Could you check a few things on this model? Use its own coordinates, in mm. Coordinates: 2 decimals unless noted, no trailing zeros. Loops run counter-clockwise (first coordinate to the right, second up) from the corner with the lowest first, then second, coordinate; pieces in that order, holes last. Notation, with made-up numbers: (-16.75, 58) - (21.25, 58) arc R24 ccw to (21.25, 83) - close; hole circle Ø7 at (14.25, 73). An arc over 180 degrees is marked (long way). Put each result on its own line as item: value. Start each with the question number.
```python
from build123d import *

# Parameters (mm, degrees)
F0_W     = 37
F0_H     = 56
F0_W_2   = 20
F0_H_2   = 20
F0_W_3   = 23
F0_H_3   = 23
F0_W_4   = 26
F0_H_4   = 18.5
F0_W_5   = 27
F0_H_5   = 3
F1_DEPTH = 1.5


with BuildPart() as f1:
    # F0 (on Top) → F1 (new body, symmetric)
    with BuildSketch(Plane.XY):
        with BuildLine():
            Line((-36.7347033552, 107.9341696352), (-246.7347033552, 107.9341696352))
            Line((-246.7347033552, 107.9341696352), (-246.7347033552, -140.0658303648))
            Line((-246.7347033552, -140.0658303648), (-36.7347033552, -140.0658303648))
            ThreePointArc((-36.7347033552, -140.0658303648), (-1.3793642959, -125.4211694242), (13.2652966448, -90.0658303648))
            Line((13.2652966448, -90.0658303648), (13.2652966448, 57.9341696352))
            ThreePointArc((13.2652966448, 57.9341696352), (-1.3793642959, 93.2895086945), (-36.7347033552, 107.9341696352))
        make_face()
        with Locations((-80.5683995187, -99.1663551629)):
            Rectangle(F0_W, F0_H, mode=Mode.SUBTRACT)
        with Locations((-43.9143308997, -91.0555796049)):
            Rectangle(F0_W_2, F0_H_2, mode=Mode.SUBTRACT)
        with Locations((-14.7307934463, -92.5555796049)):
            Rectangle(F0_W_3, F0_H_3, mode=Mode.SUBTRACT)
        with Locations((-79.3031121492, -55.4835397024)):
            Rectangle(F0_W_4, F0_H_4, mode=Mode.SUBTRACT)
        with Locations((-79.4423933029, -31.2153330278)):
            Rectangle(F0_W_4, F0_H_4, mode=Mode.SUBTRACT)
        with Locations((-43.9143308997, -55.4228818417)):
            Rectangle(F0_W_2, F0_H_2, mode=Mode.SUBTRACT)
        with Locations((-14.7307934463, -56.9228818417)):
            Rectangle(F0_W_3, F0_H_3, mode=Mode.SUBTRACT)
        with Locations((-39.8564947546, -33.6316607296)):
            Rectangle(F0_W_5, F0_H_5, mode=Mode.SUBTRACT)
        with Locations((-39.8564947546, -23.3316607296)):
            Rectangle(F0_W_5, F0_H_5, mode=Mode.SUBTRACT)
        with Locations((-7.5564947546, -33.6316607296)):
            Rectangle(F0_W_5, F0_H_5, mode=Mode.SUBTRACT)
        with Locations((-7.5564947546, -23.3316607296)):
            Rectangle(F0_W_5, F0_H_5, mode=Mode.SUBTRACT)
        with Locations((-79.4423933029, -0.9163277019)):
            Rectangle(F0_W_4, F0_H_4, mode=Mode.SUBTRACT)
        with Locations((-79.3031121492, 23.3518789727)):
            Rectangle(F0_W_4, F0_H_4, mode=Mode.SUBTRACT)
        with Locations((-39.8564947546, -8.8)):
            Rectangle(F0_W_5, F0_H_5, mode=Mode.SUBTRACT)
        with Locations((-39.8564947546, 1.5)):
            Rectangle(F0_W_5, F0_H_5, mode=Mode.SUBTRACT)
        with Locations((-7.5564947546, -8.8)):
            Rectangle(F0_W_5, F0_H_5, mode=Mode.SUBTRACT)
        with Locations((-7.5564947546, 1.5)):
            Rectangle(F0_W_5, F0_H_5, mode=Mode.SUBTRACT)
        with Locations((-43.9143308997, 23.291221112)):
            Rectangle(F0_W_2, F0_H_2, mode=Mode.SUBTRACT)
        with Locations((-14.7307934463, 24.791221112)):
            Rectangle(F0_W_3, F0_H_3, mode=Mode.SUBTRACT)
        with Locations((-80.5683995187, 67.0346944332)):
            Rectangle(F0_W, F0_H, mode=Mode.SUBTRACT)
        with Locations((-43.9143308997, 58.9239188753)):
            Rectangle(F0_W_2, F0_H_2, mode=Mode.SUBTRACT)
        with Locations((-14.7307934463, 60.4239188753)):
            Rectangle(F0_W_3, F0_H_3, mode=Mode.SUBTRACT)
    extrude(amount=F1_DEPTH, both=True)


solid = f1.part
```
(1) For pin 1 Ø0.9 at (x, z) = (-35.5, 0) entering from +Y; pin 2 Ø1.5 at (x, z) = (-18.5, 0.5) entering from -Y, each with a flat end and sliding along its axis, tell me the tip position at first contact or that it passes through.
(2) I want a section at A-A on y = -59. List the corners of the cut face in (x, z) for me, and give its area (3 significant figures).
(3) I need wall thicknesses on L1, parallel to X at y = 51.5, z = 0; L2, parallel to X at y = 25, z = -0.95; L3, parallel to Y at x = -98.5, z = 0.2. Which ranges of each line are inside material? Lowest first, please. Write a range as [from, to].
(4) I want a section at B-B on y = -109. List the corners of the cut face in (x, z) for me.
(5) I want a section at C-C on x = -45. Count the separate pieces of the cut face and the enclosed holes in it, and give its area (3 significant figures).
Answer sheet:
1. pin 1: stops at y = 107.93
1. pin 2: stops at y = -136.91
2. outline: (-246.73, -1.5) - (-92.3, -1.5) - (-92.3, 1.5) - (-246.73, 1.5) - close; (-66.3, -1.5) - (-53.91, -1.5) - (-53.91, 1.5) - (-66.3, 1.5) - close; (-33.91, -1.5) - (-26.23, -1.5) - (-26.23, 1.5) - (-33.91, 1.5) - close; (-3.23, -1.5) - (13.27, -1.5) - (13.27, 1.5) - (-3.23, 1.5) - close
2. area: 573 mm^2
3. L1: x = [-246.73, -99.07], [-62.07, -53.91], [-33.91, -26.23], [-3.23, 13.27]
3. L2: x = [-246.73, -92.3], [-66.3, -53.91], [-33.91, -26.23], [-3.23, 13.27]
3. L3: y = [-140.07, -127.17], [-71.17, 39.03], [95.03, 107.93]
4. outline: (-246.73, -1.5) - (-99.07, -1.5) - (-99.07, 1.5) - (-246.73, 1.5) - close; (-62.07, -1.5) - (9.54, -1.5) - (9.54, 1.5) - (-62.07, 1.5) - close
5. separate pieces: 9
5. enclosed holes: 0
5. area: 468 mm^2
